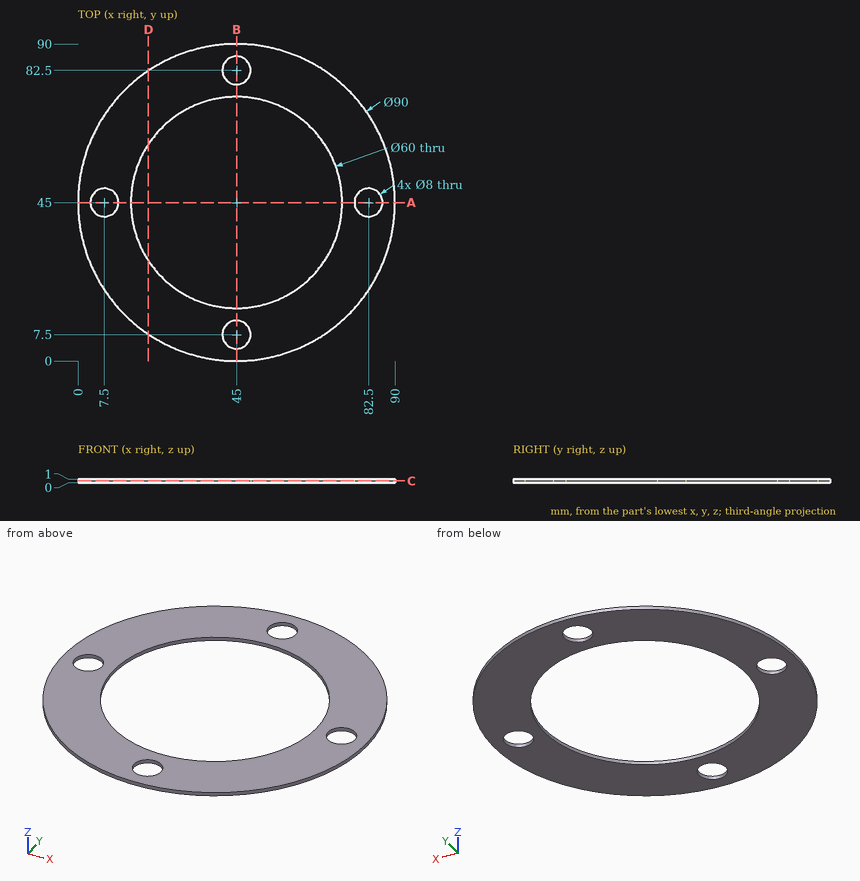
Could you check a few things on this drawing? It's one solid part, dimensions in mm from its lowest x, y, z. Round coordinates to 2 decimals unless told otherwise and drop trailing zeros. Order: outer loops, then holes, each group sorted by start corner. A loop starts at its lowest first (then second) coordinate and runs counter-clockwise, first axis right, second up.
Q1. Imagine slicing it at D-D, the plane x = 20. List the corners of the cut face in (y, z) for me, then the cut area to 3 significant figures.
Geometry says:
outline: (7.58, 0) - (28.42, 0) - (28.42, 1) - (7.58, 1) - close; (61.58, 0) - (82.42, 0) - (82.42, 1) - (61.58, 1) - close
area: 41.7 mm2
Q2. Imagine slicing it at C-C, the plane z = 0.5. List the corners of the cut face in (x, y) for me.
Geometry says:
outline: circle Ø90 at (45, 45); hole circle Ø8 at (7.5, 45); hole circle Ø60 at (45, 45); hole circle Ø8 at (45, 7.5); hole circle Ø8 at (45, 82.5); hole circle Ø8 at (82.5, 45)
Q3. Imagine slicing it at A-A, the plane y = 45. List the corners of the cut face in (x, z) for me, then the cut area to 3 significant figures.
Geometry says:
outline: (0, 0) - (3.5, 0) - (3.5, 1) - (0, 1) - close; (11.5, 0) - (15, 0) - (15, 1) - (11.5, 1) - close; (75, 0) - (78.5, 0) - (78.5, 1) - (75, 1) - close; (86.5, 0) - (90, 0) - (90, 1) - (86.5, 1) - close
area: 14.0 mm2
Q4. Please list where these lines run through material, in increasing order: probe 1 along Y at (x, z) = (7.5, 0.45); probe 2 along Y at (x, z) = (67, 0.7); probe 3 along X at (y, z) = (46, 0.4).
Geometry says:
probe 1: y = 20.13 to 41, 49 to 69.87
probe 2: y = 5.74 to 24.6, 65.4 to 84.26
probe 3: x = 0.01 to 3.63, 11.37 to 15.02, 74.98 to 78.63, 86.37 to 89.99
